Autodesk Inventor part; units mm, degrees
ref_plane "YZ Plane" through (0, 0, 0) normal (1, 0, 0) x (0, 1, 0)
ref_plane "XZ Plane" through (0, 0, 0) normal (0, 1, 0) x (-1, 0, 0)
ref_plane "XY Plane" through (0, 0, 0) normal (0, 0, 1) x (1, 0, 0)
sketch "Sketch1" plane through (0, 0, 0) normal (0, 1, 0) x (-1, 0, 0)
  line L0 (-609.6, -1219.2) -> (609.6, -1219.2)
  line L1 (609.6, -1219.2) -> (609.6, 1219.2)
  line L2 (609.6, 1219.2) -> (-609.6, 1219.2)
  line L3 (-609.6, 1219.2) -> (-609.6, -1219.2)
  line L4 (-609.6, -1219.2) -> (609.6, 1219.2) construction
  line L5 (609.6, -1219.2) -> (-609.6, 1219.2) construction
  point P0 (0, 0)
  dimension "d0" = 1219.2
  dimension "d1" = 2438.4
extrude "Extrusion1" add sketch "Sketch1" along normal blind 914.4
sketch "Sketch2" plane through (0, 914.4, 0) normal (0, 1, 0) x (1, 0, 0)
  line L0 (590.55, 1200.15) -> (-590.55, 1200.15)
  line L1 (-590.55, 1200.15) -> (-590.55, -1200.15)
  line L2 (-590.55, -1200.15) -> (590.55, -1200.15)
  line L3 (590.55, -1200.15) -> (590.55, 1200.15)
  line L4 (590.55, 1200.15) -> (-590.55, -1200.15) construction
  line L5 (-590.55, 1200.15) -> (590.55, -1200.15) construction
  point P0 (0, 0)
  dimension "d4" = 1181.1
  dimension "d5" = 2400.3
extrude "Extrusion2" cut sketch "Sketch2" against normal blind 895.35
sketch "Sketch3" plane through (0, 914.4, 0) normal (0, 1, 0) x (1, 0, 0)
  line L0 (641.35, 1250.95) -> (-641.35, 1250.95)
  line L1 (-641.35, 1250.95) -> (-641.35, -1250.95)
  line L2 (-641.35, -1250.95) -> (641.35, -1250.95)
  line L3 (641.35, -1250.95) -> (641.35, 1250.95)
  line L4 (641.35, 1250.95) -> (-641.35, -1250.95) construction
  line L5 (-641.35, 1250.95) -> (641.35, -1250.95) construction
  line L6 (-590.55, -1200.15) -> (-590.55, 1200.15)
  line L7 (590.55, 1200.15) -> (-590.55, 1200.15)
  line L8 (-590.55, 1200.15) -> (-590.55, -1200.15)
  line L9 (-590.55, -1200.15) -> (590.55, -1200.15)
  line L10 (590.55, -1200.15) -> (590.55, 1200.15)
  line L11 (590.55, 1200.15) -> (-590.55, -1200.15) construction
  line L12 (-590.55, 1200.15) -> (590.55, -1200.15) construction
  point P0 (0, 0)
  point P1 (-590.55, 1200.15)
  dimension "d8" = 1282.7
  dimension "d9" = 2501.9
extrude "Extrusion3" add sketch "Sketch3" along normal blind 31.75
pattern_linear "Rectangular Pattern1" count 2 spacing 914.4 along (0, -1, 0) of "Extrusion3"
sketch "Sketch4" plane through (-641.35, 31.75, 1250.95) normal (0, 1, 0) x (1, 0, 0)
  line L0 (0, 0) -> (1282.7, 0)
  line L1 (1282.7, 0) -> (1282.7, 76.2)
  line L2 (1282.7, 0) -> (1282.7, 2501.9)
  line L3 (1282.7, 76.2) -> (1231.9, 76.2)
  line L4 (1231.9, 2451.1) -> (1231.9, 50.8)
  line L5 (1231.9, 76.2) -> (1231.9, 50.8)
  line L6 (1231.9, 50.8) -> (1257.3, 50.8)
  line L7 (1231.9, 50.8) -> (50.8, 50.8)
  line L8 (1257.3, 50.8) -> (1257.3, 0)
  line L9 (1257.3, 0) -> (1282.7, 0)
  point P0 (641.35, 1250.95)
  point P1 (1257.3, 0)
  dimension "d15" = 76.2
  dimension "d16" = 50.8
  dimension "d17" = 25.4
  dimension "d23" = 25.4
  dimension "d24" = 50.8
  dimension "d25" = 25.4
extrude "Extrusion4" add sketch "Sketch4" along normal blind 889
mirror "Mirror2" about plane through (0, 0, 0) normal (1, 0, 0) of "Extrusion4"
mirror "Mirror3" about plane through (0, 0, 0) normal (0, 0, 1) of "Extrusion4", "Mirror2"
sketch "Sketch5" plane through (0, 946.15, 0) normal (0, 1, 0) x (1, 0, 0)
  line L0 (-590.55, -1200.15) -> (-590.55, 1200.15)
  line L1 (590.55, -695.325) -> (-590.55, -695.325)
  line L2 (-590.55, -695.325) -> (-590.55, -568.325)
  line L3 (-590.55, -568.325) -> (590.55, -568.325)
  line L4 (590.55, -568.325) -> (590.55, -695.325)
  line L5 (590.55, -695.325) -> (-590.55, -568.325) construction
  line L6 (-590.55, -695.325) -> (590.55, -568.325) construction
  line L7 (590.55, 695.325) -> (-590.55, 695.325)
  line L8 (-590.55, 695.325) -> (-590.55, 568.325)
  line L9 (-590.55, 568.325) -> (590.55, 568.325)
  line L10 (590.55, 568.325) -> (590.55, 695.325)
  line L11 (590.55, 695.325) -> (-590.55, 568.325) construction
  line L12 (-590.55, 695.325) -> (590.55, 568.325) construction
  line L13 (590.55, -63.5) -> (-590.55, -63.5)
  line L14 (-590.55, -63.5) -> (-590.55, 63.5)
  line L15 (-590.55, 63.5) -> (590.55, 63.5)
  line L16 (590.55, 63.5) -> (590.55, -63.5)
  line L17 (590.55, -63.5) -> (-590.55, 63.5) construction
  line L18 (-590.55, -63.5) -> (590.55, 63.5) construction
  line L19 (-590.55, 1200.15) -> (590.55, 1200.15)
  line L20 (590.55, -1200.15) -> (-590.55, -1200.15)
  point P0 (0, 0)
  point P1 (0, -631.825)
  point P2 (0, 631.825)
  point P3 (-590.55, -63.5)
  point P4 (-590.55, 695.325)
  dimension "d26" = 127
  dimension "d27" = 127
  dimension "d28" = 127
  dimension "d31" = 504.825
  dimension "d32" = 504.825
  dimension "d33" = 504.825
  dimension "d34" = 504.825
extrude "Extrusion5" add sketch "Sketch5" against normal blind 19.05
properties part number "CustomAquariumsTank"
Can you work these out from the model? Positions are in its coordinate system, mm. A direction names the side the tool comes from. Give positions to 0.01 mm unless a question says otherwise; leave off trailing zeros. Write each loop counter-clockwise with the first axis right and the second up, starting at its lowest first coordinate (ties: lowest second). Pieces come first, ordered by that corner, then holes. Notation, with made-up numbers: (19.5, 13.25) -> (53.5, 13.25) arc R23 ccw to (53.5, 34.25) -> close; hole circle Ø9 at (81.25, 87). An arc over 180 degrees is marked (long way). Write item = value, one per line.
(1) I need wall thicknesses on probe 1 along Y at (x, z) = (-451.5, 600.5); probe 2 along X at (y, z) = (336.5, 631.5); probe 3 along Z at (x, y) = (274, 594.5). Which ranges of each line are inside material? Lowest first, please. Write a range as from..to.
Worked out:
probe_1 = 0..19.05, 927.1..946.15
probe_2 = -609.6..-590.55, 590.55..609.6
probe_3 = -1219.2..-1200.15, 1200.15..1219.2
(2) Thinking about a two-plate mould opening in Y: for faces 4 (the face through (-615.95, 467, -1225)), 5 (the face through (-621, 471, 1250.95)), 6 (the face through (-9, 0, -18)), which applies, released by +Y, released by -Y, zero draft, split by the parting line, or undercut?
Worked out:
face_4 = undercut
face_5 = zero draft
face_6 = released by -Y
(3) Suppose I cut it at A-A on x = 119.5. Write out the boundary of the cut face in (y, z) (3 decimals).
Worked out:
outline = (0, -1250.95) -> (31.75, -1250.95) -> (31.75, -1219.2) -> (914.4, -1219.2) -> (914.4, -1250.95) -> (946.15, -1250.95) -> (946.15, -1200.15) -> (19.05, -1200.15) -> (19.05, 1200.15) -> (946.15, 1200.15) -> (946.15, 1250.95) -> (914.4, 1250.95) -> (914.4, 1219.2) -> (31.75, 1219.2) -> (31.75, 1250.95) -> (0, 1250.95) -> close; (927.1, -695.325) -> (946.15, -695.325) -> (946.15, -568.325) -> (927.1, -568.325) -> close; (927.1, -63.5) -> (946.15, -63.5) -> (946.15, 63.5) -> (927.1, 63.5) -> close; (927.1, 568.325) -> (946.15, 568.325) -> (946.15, 695.325) -> (927.1, 695.325) -> close
(4) Suppose I cut it at D-D on z = 882.5. Write out the boundary of the cut face in (x, y), then the cut area to 3 significant figures.
Worked out:
outline = (-641.35, 0) -> (641.35, 0) -> (641.35, 31.75) -> (609.6, 31.75) -> (609.6, 914.4) -> (641.35, 914.4) -> (641.35, 946.15) -> (590.55, 946.15) -> (590.55, 19.05) -> (-590.55, 19.05) -> (-590.55, 946.15) -> (-641.35, 946.15) -> (-641.35, 914.4) -> (-609.6, 914.4) -> (-609.6, 31.75) -> (-641.35, 31.75) -> close
area = 62,600 mm^2
(5) I'm going to push flat-ended pins straight in: P1, Ø5, axis at y = 425, z = 284.5, coming from the +X side; P2, Ø5, axis at y = 97, z = 340.5, coming from the -X side; P3, Ø3, axis at x = -613, y = 688.5, coming from the -Z side. Where does each tip first touch, or does it pass through?
Worked out:
P1 = 609.6
P2 = -609.6
P3 = -1200.15
(6) Suppose I cut it at C-C on z = 13. Write out the boundary of the cut face in (x, y), then the cut area to 3 significant figures.
Worked out:
outline = (-641.35, 0) -> (641.35, 0) -> (641.35, 31.75) -> (609.6, 31.75) -> (609.6, 914.4) -> (641.35, 914.4) -> (641.35, 946.15) -> (-641.35, 946.15) -> (-641.35, 914.4) -> (-609.6, 914.4) -> (-609.6, 31.75) -> (-641.35, 31.75) -> close; hole (-590.55, 19.05) -> (590.55, 19.05) -> (590.55, 927.1) -> (-590.55, 927.1) -> close
area = 85,100 mm^2
(7) For faces 1 (the face through (615.95, 467, 1225)), 2 (the face through (-8, 927.1, 631)), 3 (the face through (9, 467, -1219.2)), which set-ups out of +Z, -Z, +X, -X, +Y, -Y let a thin tool reach every point of the face, with its end or its side?
Worked out:
face_1 = +Z
face_2 = none
face_3 = -Z
